```python
from build123d import *

# Parameters (mm, degrees)
F0_R     = 14.2875
F1_DEPTH = 3.175
F2_R     = 3.175
F3_DEPTH = 25.4
F5_DEPTH = 25.4


with BuildPart() as f1:
    # F0 (on Right) → F1 (new body)
    with BuildSketch(Plane.YZ):
        with BuildLine():
            Line((-190.5, -25.4), (12.7, -25.4))
            ThreePointArc((12.7, -25.4), (21.680256, -21.680256), (25.4, -12.7))
            Line((25.4, -12.7), (25.4, 12.7))
            ThreePointArc((25.4, 12.7), (21.680256, 21.680256), (12.7, 25.4))
            Line((12.7, 25.4), (0, 25.4))
            ThreePointArc((0, 25.4), (-23.400478, 30.227273), (-43.360512, 43.360512))
            Line((-43.360512, 43.360512), (-143.684098, 143.684098))
            ThreePointArc((-143.684098, 143.684098), (-187.732321, 77.761273), (-203.2, 0))
            Line((-203.2, 0), (-203.2, -12.7))
            ThreePointArc((-203.2, -12.7), (-199.480256, -21.680256), (-190.5, -25.4))
        make_face()
        Circle(F0_R, mode=Mode.SUBTRACT)
    extrude(amount=F1_DEPTH)

    # F2 (on face) → F3 (cut)
    with BuildSketch(Plane.YZ.offset(3.175)):
        with Locations((-192.993104, -16.237834)):
            Circle(F2_R)
        with Locations((-193.458162, 9.162166)):
            Circle(F2_R)
        with Locations((-147.064992, 126.023386)):
            Circle(F2_R)
        with Locations((-162.292342, 105.693904)):
            Circle(F2_R)
        with Locations((-174.728316, 83.546522)):
            Circle(F2_R)
        with Locations((-184.159019, 59.962166)):
            Circle(F2_R)
        with Locations((-190.566163, 34.562166)):
            Circle(F2_R)
    extrude(amount=-F3_DEPTH, mode=Mode.SUBTRACT)

    # F4 (on face) → F5 (cut)
    with BuildSketch(Plane.YZ.offset(3.175)):
        with BuildLine():
            ThreePointArc((-52.430116, 31.489606), (-55.287221, 32.673058), (-57.16982, 30.219606))
            Line((-57.16982, 30.219606), (-57.16982, -10.16))
            ThreePointArc((-57.16982, -10.16), (-56.425871, -11.956051), (-54.62982, -12.7))
            Line((-54.62982, -12.7), (-31.316644, -12.7))
            ThreePointArc((-31.316644, -12.7), (-29.116939, -11.43), (-29.116939, -8.89))
            Line((-29.116939, -8.89), (-52.430116, 31.489606))
        make_face()
        with BuildLine():
            ThreePointArc((-72.40982, -12.7), (-70.613769, -11.956051), (-69.86982, -10.16))
            Line((-69.86982, -10.16), (-69.86982, 30.219606))
            ThreePointArc((-69.86982, 30.219606), (-71.75242, 32.673058), (-74.609525, 31.489606))
            Line((-74.609525, 31.489606), (-97.922701, -8.89))
            ThreePointArc((-97.922701, -8.89), (-97.922701, -11.43), (-95.722997, -12.7))
            Line((-95.722997, -12.7), (-72.40982, -12.7))
        make_face()
        with BuildLine():
            ThreePointArc((-114.787103, -3.220591), (-112.904503, -5.674043), (-110.047398, -4.490591))
            Line((-110.047398, -4.490591), (-86.734222, 35.889015))
            ThreePointArc((-86.734222, 35.889015), (-86.734222, 38.429015), (-88.933926, 39.699015))
            Line((-88.933926, 39.699015), (-112.247103, 39.699015))
            ThreePointArc((-112.247103, 39.699015), (-114.043154, 38.955067), (-114.787103, 37.159015))
            Line((-114.787103, 37.159015), (-114.787103, -3.220591))
        make_face()
        with BuildLine():
            Line((-127.487103, -10.16), (-127.487103, 30.219606))
            ThreePointArc((-127.487103, 30.219606), (-129.369702, 32.673058), (-132.226807, 31.489606))
            Line((-132.226807, 31.489606), (-155.539984, -8.89))
            ThreePointArc((-155.539984, -8.89), (-155.539984, -11.43), (-153.340279, -12.7))
            Line((-153.340279, -12.7), (-130.027103, -12.7))
            ThreePointArc((-130.027103, -12.7), (-128.231051, -11.956051), (-127.487103, -10.16))
        make_face()
        with BuildLine():
            ThreePointArc((-169.229385, 39.699015), (-171.474449, 38.769079), (-172.404385, 36.524015))
            Line((-172.404385, 36.524015), (-172.404385, -3.220591))
            ThreePointArc((-172.404385, -3.220591), (-170.521786, -5.674043), (-167.664681, -4.490591))
            Line((-167.664681, -4.490591), (-144.351504, 35.889015))
            ThreePointArc((-144.351504, 35.889015), (-144.351504, 38.429015), (-146.551209, 39.699015))
            Line((-146.551209, 39.699015), (-169.229385, 39.699015))
        make_face()
        with BuildLine():
            Line((-162.496961, 76.890181), (-174.454135, 56.210428))
            ThreePointArc((-174.454135, 56.210428), (-174.455359, 53.669722), (-172.255247, 52.399015))
            Line((-172.255247, 52.399015), (-162.435202, 52.399015))
            ThreePointArc((-162.435202, 52.399015), (-160.63915, 53.142964), (-159.895202, 54.939015))
            Line((-159.895202, 54.939015), (-159.895202, 76.192146))
            ThreePointArc((-159.895202, 76.192146), (-160.92836, 77.539032), (-162.496961, 76.890181))
        make_face()
        with BuildLine():
            ThreePointArc((-142.3178, 79.023671), (-145.162448, 80.518448), (-147.195202, 78.029613))
            Line((-147.195202, 78.029613), (-147.195202, 54.939015))
            ThreePointArc((-147.195202, 54.939015), (-146.451253, 53.142964), (-144.655202, 52.399015))
            Line((-144.655202, 52.399015), (-134.835156, 52.399015))
            ThreePointArc((-134.835156, 52.399015), (-132.716607, 53.537821), (-132.497754, 55.933073))
            Line((-132.497754, 55.933073), (-142.3178, 79.023671))
        make_face()
        with BuildLine():
            ThreePointArc((-127.205028, 81.389885), (-129.323578, 80.25108), (-129.54243, 77.855827))
            Line((-129.54243, 77.855827), (-119.722385, 54.765229))
            ThreePointArc((-119.722385, 54.765229), (-116.877736, 53.270452), (-114.844983, 55.759288))
            Line((-114.844983, 55.759288), (-114.844983, 78.849885))
            ThreePointArc((-114.844983, 78.849885), (-115.588931, 80.645936), (-117.384983, 81.389885))
            Line((-117.384983, 81.389885), (-127.205028, 81.389885))
        make_face()
        with BuildLine():
            Line((-104.493987, 80.426647), (-104.493987, 54.939015))
            ThreePointArc((-104.493987, 54.939015), (-103.750038, 53.142964), (-101.953987, 52.399015))
            Line((-101.953987, 52.399015), (-76.188018, 52.399015))
            ThreePointArc((-76.188018, 52.399015), (-73.838733, 53.973375), (-74.401746, 56.744794))
            Line((-74.401746, 56.744794), (-100.167715, 82.232425))
            ThreePointArc((-100.167715, 82.232425), (-102.932371, 82.770653), (-104.493987, 80.426647))
        make_face()
        with BuildLine():
            Line((-153.851107, 94.089885), (-118.334172, 94.089885))
            ThreePointArc((-118.334172, 94.089885), (-115.984887, 95.664245), (-116.5479, 98.435663))
            Line((-116.5479, 98.435663), (-136.720031, 118.389885))
            ThreePointArc((-136.720031, 118.389885), (-138.677975, 119.118298), (-140.519792, 118.13248))
            Line((-140.519792, 118.13248), (-155.864596, 98.178259))
            ThreePointArc((-155.864596, 98.178259), (-156.129755, 95.507671), (-153.851107, 94.089885))
        make_face()
    extrude(amount=-F5_DEPTH, mode=Mode.SUBTRACT)


solid = f1.part
```
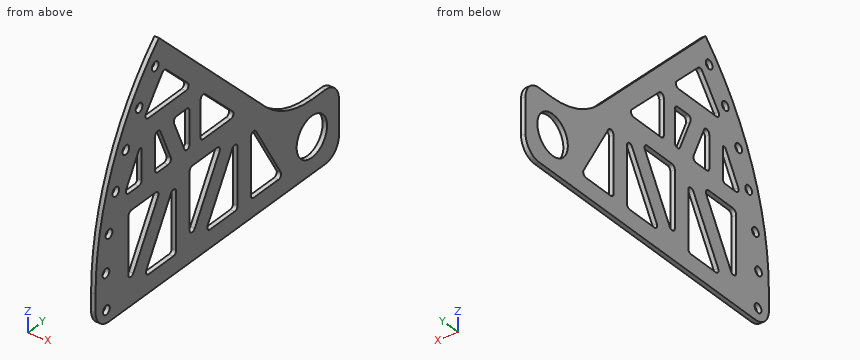
Check sheet for the modelled part. Datum: model origin and axes. Units: mm. Round coordinates to 2 decimals unless told otherwise and drop trailing zeros. Loops run counter-clockwise (first coordinate to the right, second up) from the corner with the lowest first, then second, coordinate; pieces in that order, holes last. Notation, with made-up numbers: (60.5, 71.25) - (92.5, 71.25) arc R19 cw to (92.5, 98.25) - close; hole circle Ø4 at (-22, 13). An arc over 180 degrees is marked (long way). Write item = value, one per line. Start each with the question number.
Q1. Section check B-B (y = -93). Record the boundary of the cut face in (x, z) (3 decimals), plus the area to 3 significant figures.
Q2. Depth check by flat-ended pin: P1, Ø1, axis at x = 1.5, z = 65, coming from the -Y side; P2, Ø1.6, axis at x = 1, z = 19.5, coming from the +Y side. Enter the tip coordinate at first touch or a pass-through.
Q3. Thickness scan on L1, parallel to Y at x = 1.45, z = 53.5; L2, parallel to Y at x = 1.4, z = 31; L3, parallel to Y at x = 2.8, z = 106. Record the ranges inside material, lowest first.
Q4. Section check A-A (y = 4.5). Record the boundary of the cut face in (x, z) (3 decimals), plus the area to 3 significant figures.
Q5. Section check C-C (x = 2). Count the separate pieces of the cut face and the enclosed holes in it, plus the area to 3 significant figures.
Derived:
q1.outline = (0, -25.4) - (3.175, -25.4) - (3.175, -12.7) - (0, -12.7) - close; (0, -0.364) - (3.175, -0.364) - (3.175, 25.036) - (0, 25.036) - close; (0, 39.699) - (3.175, 39.699) - (3.175, 52.399) - (0, 52.399) - close; (0, 75.142) - (3.175, 75.142) - (3.175, 93) - (0, 93) - close
q1.area = 218 mm^2
q2.P1 = -192.69
q2.P2 = 23.89
q3.L1 = -196.03 to -174.35, -160.34 to -146.75, -132.74 to -118.55, -116.22 to -104.05, -74.09 to -53.5
q3.L2 = -200.82 to -172.4, -147.17 to -132.51, -127.61 to -114.79, -89.56 to -74.89, -69.99 to -57.05, -52.15 to -25.19
q3.L3 = -173.36 to -165.45, -159.13 to -149.85, -124.19 to -106
q4.outline = (0, -25.4) - (3.175, -25.4) - (3.175, -13.56) - (0, -13.56) - close; (0, 13.56) - (3.175, 13.56) - (3.175, 25.4) - (0, 25.4) - close
q4.area = 75.2 mm^2
q5.separate_pieces = 1
q5.enclosed_holes = 18
q5.area = 16,300 mm^2
